```python
from build123d import *

# Parameters (mm, degrees)
FILLET_1_R     = 0.3
CHAMFER_1_SIZE = 0.5
FILLET_2_R     = 0.1


with BuildPart() as part:
    # Эскиз18 → Повернуть1 (revolve)
    with BuildSketch(Plane(origin=(0, 0, 0), x_dir=(0, 0, -1), z_dir=(1, 0, 0)), mode=Mode.PRIVATE) as revolve_1_sk:
        Polygon((-10, -15), (-6, -15), (-6, -14), (-4, -14), (-4, -15), (0, -15), (0, -17), (-4.5, -17), (-4.5, -16), (-5.5, -16), (-5.5, -17), (-10, -17), align=None)
    revolve(revolve_1_sk.sketch.rotate(Axis((0, 0, 0), (0, 0, 1)), 270), axis=Axis((0, 0, 0), (0, 0, 1)))

    # Скругление1
    fillet_1_edges = [part.edges().sort_by_distance(p)[0] for p in [
        (16, 0, 5.5),
        (16, 0, 4.5),
    ]]
    fillet(fillet_1_edges, radius=FILLET_1_R)

    # Фаска1
    chamfer_1_edges = [part.edges().sort_by_distance(p)[0] for p in [
        (17, 0, 0),
        (17, 0, 10),
        (17, 0, 5.5),
        (17, 0, 4.5),
    ]]
    chamfer(chamfer_1_edges, length=CHAMFER_1_SIZE)

    # Скругление2
    fillet_2_edges = [part.edges().sort_by_distance(p)[0] for p in [
        (15, 0, 4),
        (15, 0, 6),
    ]]
    fillet(fillet_2_edges, radius=FILLET_2_R)


solid = part.part
```
Can you work these out from the model? Positions are in its coordinate system, mm. A direction names the side the tool comes from. Coordinates: 2 decimals unless noted, no trailing zeros. Write each loop counter-clockwise with the first axis right and the second up, starting at its lowest first coordinate (ties: lowest second). Pieces come first, ordered by that corner, then holes. Notation, with made-up numbers: (21, 23.25) - (66, 23.25) arc R21 ccw to (66, 45.25) - close; hole circle Ø3 at (-27, -1). An arc over 180 degrees is marked (long way). Return JSON: item names as keys, results as strings.
Q1. Thinking about a two-plate mould opening in Y: for faces 5 (the cylindrical face through (2.213, -16.855, 2.274)), 6 (the cylindrical face through (3.03, 13.67, 4.99)), 7 (the flat face through (9, 11, 4)), 8 (the flat face through (4, 15, 0)), which applies, +Y half, -Y half, draft (parallel to the pull), parting line (faces both ways), or undercut?
Computed values:
{"face 5": "parting line", "face 6": "undercut", "face 7": "undercut", "face 8": "draft"}
Q2. I'm going to push flat-ended pins straight in: pin 1 Ø1 at (x, z) = (6, 7.5) entering from -Y; pin 2 Ø16.5 at (x, y) = (7, 1.5) entering from +Z; pin 3 Ø5 at (x, z) = (-13, 5) entering from +Y; pin 4 Ø10 at (x, y) = (3, 3.5) entering from -Z. Where does each tip first touch, or does it pass through?
Computed values:
{"pin 1": "stops at y = -16.09", "pin 2": "stops at z = 10", "pin 3": "stops at y = 13.2", "pin 4": "passes through"}
Q3. On a 3-axis mill with a long thin cutter (end or side, diameter ignored), from which of +Z, -Z, +X, -X, +Y, -Y can I reach the whole of each face in a straight line? I mean faces 1 (the cylindrical face through (14.985, -0.66, 1.923)), 2 (the cylindrical face through (3.47, 15.62, 5)), 3 (the cylindrical face through (14.985, -0.66, 8.023)), 4 (the cylindrical face through (2.213, -16.855, 7.774)). Say none if no direction works.
Computed values:
{"face 1": "-Z", "face 2": "none", "face 3": "+Z", "face 4": "+Z, -Z"}
Q4. If we section it at A-A (z = 2.5): Please give me the cut outline in (x, y), then the cut area to 3 significant figures.
Computed values:
{"outline": "circle Ø34 at (0, 0); hole circle Ø30 at (0, 0)", "area": "201 mm2"}
Q5. Please list where these lines run through material, in increasing order: L1, parallel to Y at x = 0, z = 7.7; L2, parallel to Z at x = -3, y = 16; L3, parallel to X at y = 3.5, z = 1.5. Write a range as from..to.
Computed values:
{"L1": "y = -17..-15, 15..17", "L2": "z = 0..4.5, 5.5..10", "L3": "x = -16.64..-14.59, 14.59..16.64"}
